Here's how the part is built. I have some questions about the finished solid (model axes, mm). Face numbers are marked on the shaded views. A direction names the side the tool comes from. Round coordinates to 2 decimals unless told otherwise and drop trailing zeros. Write each loop counter-clockwise with the first axis right and the second up, starting at its lowest first coordinate (ties: lowest second). Pieces come first, ordered by that corner, then holes. Notation, with made-up numbers: (59, -32.5) -> (83, -32.5) arc R31 cw to (83, -6.5) -> close; hole circle Ø10 at (67.25, 77.5). An arc over 180 degrees is marked (long way). Put each result on its own line as item: value. Start each with the question number.
1) We'd pull the mould along Z, two halves only. Please class the marked faces 1, 2 and 3: released by +Z, released by -Z, zero draft, split by the parting line, or undercut.
2) I want a section at A-A, the plane x = -13. List the corners of the cut face in (y, z) for me.
3) Will these pins go through, and if not, where does the flat tip stop? P1, Ø6, axis at y = 6.5, z = -5, coming from the -X side; P2, Ø6.5, axis at y = 6, z = -6.92, coming from the -X side; P3, Ø1.6, axis at y = 6, z = -13.5, coming from the +X side.
4) If I drill on line 1 along Z through (x, y) = (-6.5, 9); line 2 along X through (y, z) = (2.25, -6.25); line 3 along Z through (x, y) = (-7.5, 6.25), over which ranges is the centre line in solid material (lowest first)? Write a range as [from, to].
5) I want a section at B-B, the plane z = 6.5. List the corners of the cut face in (x, y) for me.
6) I want a section at C-C, the plane y = 6.25. Give the number of separate pieces and of enclosed holes in the cut face, then the cut area to 3 significant figures.
7) Which directions (+Z, -Z, +X, -X, +Y, -Y) give clear straight access to the entire face, cutting with the end or side of a thin tool? Please do the marked faces 4, 5, 6 and 7.
from build123d import *

# Parameters (mm, degrees)
SKETCH2_W           = 10
SKETCH2_H           = 20
BOSS_EXTRUDE1_DEPTH = 12
SKETCH4_R           = 1.45
CUT_EXTRUDE1_DEPTH  = 22
SKETCH5_R           = 0.201375714
CUT_EXTRUDE2_DEPTH  = 34
SKETCH6_R           = 4
CUT_EXTRUDE3_DEPTH  = 2
SKETCH7_W           = 2
SKETCH7_H           = 12
BOSS_EXTRUDE4_DEPTH = 2
CHAMFER1_SIZE       = 1


with BuildPart() as part:
    # Sketch2 → Boss-Extrude1 (new body)
    with BuildSketch(Plane(origin=(0, 0, 0), x_dir=(1, 0, 0), z_dir=(0, 1, 0))):
        with Locations((-9.742268041, 1.958762887)):
            Rectangle(SKETCH2_W, SKETCH2_H)
    extrude(amount=BOSS_EXTRUDE1_DEPTH)

    # Sketch4 → Cut-Extrude1 (cut)
    with BuildSketch(Plane(origin=(0, 12, 0), x_dir=(1, 0, 0), z_dir=(0, 1, 0))):
        with Locations(Location((-12.161364559, -5.505377828, 0), (0, 0, 270))):
            Circle(SKETCH4_R)
    extrude(amount=-CUT_EXTRUDE1_DEPTH, mode=Mode.SUBTRACT)

    # Sketch5 → Cut-Extrude2 (cut)
    # profile 1 of 2: a face of its own
    with BuildSketch(Plane.XZ):
        with BuildLine():
            Line((-6.242268041, -9.519810645), (-6.242268041, 2.231313467))
            ThreePointArc((-6.242268041, 2.231313467), (-6.418660257, 2.371807213), (-6.642496519, 2.344420462))
            add(Edge.make_bspline(
                [(-6.642496519, 2.344420462), (-6.66140925, 2.33038701), (-6.68025518, 2.316351489), (-6.699034308, 2.302313899)],
                knots=[0.023195247, 0.023195247, 0.023195247, 0.023195247, 0.026563492, 0.026563492, 0.026563492, 0.026563492], degree=3))
            add(Edge.make_bspline(
                [(-6.699034308, 2.302313899), (-9.211405567, 0.424290628), (-10.573371912, -1.556580292), (-10.656105812, -3.577082439), (-10.65744251, -3.644248589)],
                knots=[0.026563492, 0.026563492, 0.026563492, 0.026563492, 0.477185204, 0.492669554, 0.492669554, 0.492669554, 0.492669554], degree=3))
            add(Edge.make_bspline(
                [(-6.699034308, -9.590811077), (-9.211405567, -7.712787806), (-10.573371912, -5.731916886), (-10.656105812, -3.711414739), (-10.65744251, -3.644248589)],
                knots=[0.026563492, 0.026563492, 0.026563492, 0.026563492, 0.477185204, 0.492669554, 0.492669554, 0.492669554, 0.492669554], degree=3))
            add(Edge.make_bspline(
                [(-6.642496519, -9.63291764), (-6.66140925, -9.618884188), (-6.68025518, -9.604848667), (-6.699034308, -9.590811077)],
                knots=[0.023195247, 0.023195247, 0.023195247, 0.023195247, 0.026563492, 0.026563492, 0.026563492, 0.026563492], degree=3))
            ThreePointArc((-6.642496519, -9.63291764), (-6.418660257, -9.660304391), (-6.242268041, -9.519810645))
        make_face()
        with Locations((-7.81457768, -3.845615826)):
            Circle(SKETCH5_R, mode=Mode.SUBTRACT)
    # profile 2 of 2: a face of its own
    with BuildSketch(Plane.XZ):
        with Locations((-7.81457768, -3.845615826)):
            Circle(SKETCH5_R)
    extrude(amount=-CUT_EXTRUDE2_DEPTH, mode=Mode.SUBTRACT)

    # Sketch6 → Cut-Extrude3 (cut)
    with BuildSketch(Plane.ZY.offset(14.742268041)):
        with Locations((-6.916385821, 6)):
            Circle(SKETCH6_R)
    extrude(amount=-CUT_EXTRUDE3_DEPTH, mode=Mode.SUBTRACT)

    # Sketch7 → Boss-Extrude4 (add)
    with BuildSketch(Plane(origin=(0, 0, -11.958762887), x_dir=(-1, 0, 0), z_dir=(0, 0, -1))):
        with Locations((13.742268041, 6)):
            Rectangle(SKETCH7_W, SKETCH7_H)
    extrude(amount=BOSS_EXTRUDE4_DEPTH)

    # Chamfer1
    chamfer1_edges = [part.edges().sort_by_distance(p)[0] for p in [
        (-4.742268041, 0, -1.958762887),
        (-4.742268041, 12, -1.958762887),
    ]]
    chamfer(chamfer1_edges, length=CHAMFER1_SIZE)


solid = part.part
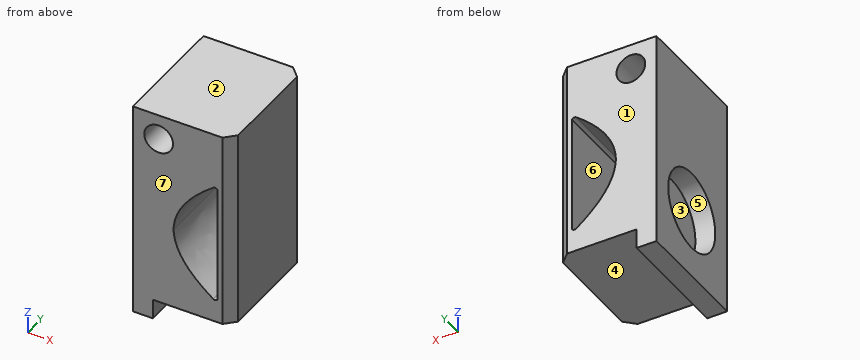
Findings:
1. face 1: zero draft
1. face 2: released by +Z
1. face 3: undercut
2. outline: (0, -13.96) -> (12, -13.96) -> (12, 4.32) -> (0, 4.32) -> close; (0, 6.69) -> (12, 6.69) -> (12, 8.04) -> (0, 8.04) -> close; hole circle Ø8 at (6, -6.92)
3. P1: stops at x = -14.74
3. P2: stops at x = -12.74
3. P3: stops at x = -12.74
4. line 1: z = [-11.96, -9.67], [2.38, 8.04]
4. line 2: x = [-12.74, -9.88], [-6.24, -4.74]
4. line 3: z = [-11.96, -8.96], [1.67, 8.04]
5. outline: (-14.74, 0) -> (-13.22, 0) -> (-13.22, 12) -> (-14.74, 12) -> close; (-11.11, 0) -> (-5.74, 0) -> (-4.74, 1) -> (-4.74, 11) -> (-5.74, 12) -> (-11.11, 12) -> close
6. separate pieces: 1
6. enclosed holes: 2
6. area: 145 mm2
7. face 4: -Z, +X, +Y, -Y
7. face 5: -X
7. face 6: +Y, -Y
7. face 7: +Z, -Z, +X, -X, -Y
